Could you check a few things on this model? Use its own coordinates, in mm. Face numbers are marked on the shaded views. A direction names the side the tool comes from. Round coordinates to 2 decimals unless told otherwise and drop trailing zeros. Order: outer loops, then holes, each group sorted by start corner. A loop starts at its lowest first (then second) coordinate and runs counter-clockwise, first axis right, second up. Notation, with made-up numbers: (14, -37) - (26, -37) arc R5 ccw to (26, -28) - close; hole circle Ø11 at (68.5, -22.5). An arc over 180 degrees is marked (long way). Use one line per item in the form item = value.
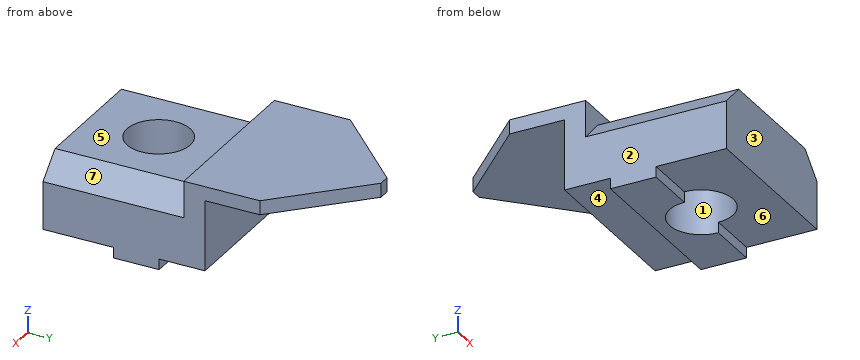
from build123d import *

# Parameters (mm, degrees)
F0_W      = 76.2
F0_H      = 31.75
F0_H_2    = 4.7625
F1_DEPTH  = 133.35
F2_SIZE   = 10.16
F0_H_3    = 6.35
F3_DEPTH  = 9.525
F4_DEPTH  = 69.85
F6_DEPTH  = 51.308
F7_SIZE2  = 35.56
F7_SIZE   = 35.56
F8_R      = 14.2875
F9_DEPTH  = 39.116
F10_DEPTH = 9.525
F11_W     = 20.6375
F11_H     = 4.7625
F11_W_2   = 31.75
F12_DEPTH = 84.836


with BuildPart() as f1:
    # F0 (on Front) → F1 (new body)
    with BuildSketch(Plane.XZ):
        with Locations((-18.9479482412, -5.8624097556)):
            Rectangle(F0_W, F0_H)
        with Locations((-18.9479482412, -24.1186597556)):
            Rectangle(F0_W, F0_H_2)
    extrude(amount=F1_DEPTH)

    # F2
    f2_edges = [f1.edges().sort_by_distance(p)[0] for p in [
        (19.152052, -66.675, 10.01259),
        (-57.047948, -66.675, 10.01259),
    ]]
    chamfer(f2_edges, length=F2_SIZE)

    # F0 (on Front) → F3 (join)
    with BuildSketch(Plane.XZ):
        with Locations((-18.9479482412, -5.8624097556)):
            Rectangle(F0_W, F0_H)
        with Locations((-18.9479482412, 13.1875902444)):
            Rectangle(F0_W, F0_H_3)
    extrude(amount=-F3_DEPTH)

    # F0 (on Front) → F4 (join)
    with BuildSketch(Plane.XZ):
        with Locations((-18.9479482412, 13.1875902444)):
            Rectangle(F0_W, F0_H_3)
    extrude(amount=-F4_DEPTH)

    # F5 (on face) → F6 (cut)
    with BuildSketch(Plane.XY.offset(10.0125902444)):
        Polygon((8.9920517588, -63.5), (-46.8879482412, -63.5), (-73.6699253321, -63.5), (-73.6699253321, -133.35), (35.7825346291, -133.35), (35.7825346291, -63.5), align=None)
    extrude(amount=-F6_DEPTH, mode=Mode.SUBTRACT)

    # F7
    f7_edges = [f1.edges().sort_by_distance(p)[0] for p in [
        (-57.047948, 69.85, 13.18759),
        (19.152052, 69.85, 13.18759),
    ]]
    chamfer(f7_edges, length=F7_SIZE, length2=F7_SIZE2)

    # F8 (on face) → F9 (cut)
    with BuildSketch(Plane.XY.offset(10.0125902444)):
        with Locations((-18.9479482412, -31.75)):
            Circle(F8_R)
    extrude(amount=-F9_DEPTH, mode=Mode.SUBTRACT)

    # F10 (add): a face of the model
    f10_faces = [f1.faces().sort_by_distance(p)[0] for p in [
        (-18.9479482412, 0, -24.1186597556),
    ]]
    extrude(f10_faces, amount=F10_DEPTH)

    # F11 (on face) → F12 (cut)
    with BuildSketch(Plane(origin=(-57.0479482412, 0, 0), x_dir=(0, -1, 0), z_dir=(-1, 0, 0))):
        with Locations((0.79375, -24.1186597556)):
            Rectangle(F11_W, F11_H)
        with Locations((47.625, -24.1186597556)):
            Rectangle(F11_W_2, F11_H)
    extrude(amount=-F12_DEPTH, mode=Mode.SUBTRACT)


solid = f1.part
Item 1: Imagine slicing it at B-B on y = -30. Please give me the cut outline in (x, z), plus the area to 3 significant figures.
Found:
outline = (-57.05, -26.5) - (-33.13, -26.5) - (-33.13, 10.01) - (-46.89, 10.01) - (-57.05, -0.15) - close; (-4.77, -26.5) - (19.15, -26.5) - (19.15, -0.15) - (8.99, 10.01) - (-4.77, 10.01) - close
area = 1,640 mm2
Item 2: I need wall thicknesses on L1, parallel to X at y = -31.75, z = -1.5; L2, parallel to Z at x = -37.5, y = -52.5; L3, parallel to Z at x = -53, y = 4.5. Which ranges of each line are inside material? Lowest first, please.
Found:
L1 = -57.05 to -33.24, -4.66 to 19.15
L2 = -21.74 to 10.01
L3 = -21.74 to 16.36
Item 3: For the marked faces 4, 5, 6 and 7, which set-ups out of +Z, -Z, +X, -X, +Y, -Y let a thin tool reach every point of the face, with its end or its side?
Found:
face_4 = -Z, +X, -X, +Y
face_5 = +Z, +X, -X, -Y
face_6 = -Z, +X, -X, -Y
face_7 = +Z, +X, -Y
Item 4: Imagine slicing it at C-C on x = -7.5. Please give me the cut outline in (y, z) (1 decimal), plus the area to 3 significant figures.
Found:
outline = (-63.5, -21.7) - (-40.3, -21.7) - (-40.3, 10) - (-63.5, 10) - close; (-23.2, -26.5) - (-11.1, -26.5) - (-11.1, -21.7) - (9.5, -21.7) - (9.5, 10) - (60.9, 10) - (60.9, 16.4) - (0, 16.4) - (0, 10) - (-23.2, 10) - close
area = 2,220 mm2
Item 5: Will these pins go through, and if not, where does the flat tip stop? P1, Ø1.4, axis at x = -20.5, z = -25, coming from the +Y side; P2, Ø10, axis at y = -31, z = 7, coming from the -X side; P3, Ø2, axis at x = -13.5, y = 4, coming from the -Z side.
Found:
P1 = -11.11
P2 = -54.9
P3 = -21.74
Item 6: Imagine slicing it at D-D on z = 11.5. Please give me the cut outline in (x, y).
Found:
outline = (-57.05, 0) - (19.15, 0) - (19.15, 34.29) - (-16.41, 69.85) - (-21.49, 69.85) - (-57.05, 34.29) - close
Item 7: If we mould it in two halves opening along Y, with no side actions, what happens to the marked faces 1, 2 and 3? For each: released by +Y, released by -Y, zero draft, split by the parting line, or undercut.
Found:
face_1 = undercut
face_2 = zero draft
face_3 = released by -Y
